Here's how the part is built. I have some questions about the finished solid (model axes, mm). A direction names the side the tool comes from. Round coordinates to 2 decimals unless told otherwise and drop trailing zeros. Write each loop counter-clockwise with the first axis right and the second up, starting at its lowest first coordinate (ties: lowest second). Pieces come first, ordered by that corner, then holes. Notation, with made-up numbers: (50, 28.25) -> (99, 28.25) arc R16 cw to (99, 32.25) -> close; hole circle Ø9 at (81.25, 34.25). An arc over 180 degrees is marked (long way). Put each result on its own line as item: value. Start each with the question number.
1. Suppose I cut it at C-C (x = 0). Please give me the cut outline in (y, z), then the cut area to 3 significant figures.
2. Suppose I cut it at D-D (x = 4). Please give me the cut outline in (y, z), then the cut area to 3 significant figures.
3. Suppose I cut it at B-B (y = 2.75). Please give me the cut outline in (x, z), then the cut area to 3 significant figures.
4. We'd pull the mould along Y, two halves only. Please class faces 4 (the face through (0.07, 2.95, 29.48)), 5 (the face through (5, 0.7, 22)), 6 (the face through (2, 0, 14)), 7 (the face through (0.07, 5.77, 29.56)): +Y half, -Y half, draft (parallel to the pull), parting line (faces both ways), or undercut.
5. Suppose I cut it at A-A (z = 5). Please give me the cut outline in (x, y).
6. For pin 1 (4 mm diameter, centred on x = -3, y = 6, fed in from +Z); pin 2 (5 mm diameter, centred on x = 0, z = 15, fed in from +Y), each with a flat end and sliding along its axis, tell me the tip position at first contact or that it passes through.
7. I need wall thicknesses on probe 1 along X at (y, z) = (0.3, 5); probe 2 along Y at (x, z) = (0.5, 12); probe 3 along Z at (x, y) = (-3.75, 5.25). Which ranges of each line are inside material? Lowest first, please. Write a range as from..to.
8. Which directions (+Z, -Z, +X, -X, +Y, -Y) give clear straight access to the entire face, cutting with the end or side of a thin tool? Please do faces 1 (the face through (0.07, 2.951, 35.613)), 2 (the face through (0, 0.5, 0)), 3 (the face through (0.07, 2.829, 28.486)).
```python
from build123d import *

# Parameters (mm, degrees)
EXTRUDE_THIN1_DEPTH = 5
FILLET1_R           = 3
SKETCH2_R           = 1.5
CUT_EXTRUDE1_DEPTH  = 10


with BuildPart() as part:
    # Sketch1 → Extrude-Thin1 (new, symmetric)
    with BuildSketch(Plane(origin=(0, 0, 0), x_dir=(0, 0, -1), z_dir=(1, 0, 0))):
        with BuildLine():
            Line((0, 0), (-28.808246407, 0))
            ThreePointArc((-28.808246407, 0), (-29.574290851, 0.35721239), (-29.79305416, 1.173648178))
            Line((-29.79305416, 1.173648178), (-29.156852475, 4.781727229))
            ThreePointArc((-29.156852475, 4.781727229), (-29.568083792, 5.774527451), (-30.641660228, 5.821400811))
            Line((-30.641660228, 5.821400811), (-40.724622204, 0))
            Line((-40.724622204, 0), (-41.224622204, 0.866025404))
            Line((-41.224622204, 0.866025404), (-31.141660228, 6.687426215))
            ThreePointArc((-31.141660228, 6.687426215), (-28.994507355, 6.593679496), (-28.172044722, 4.608079052))
            Line((-28.172044722, 4.608079052), (-28.808246407, 1))
            Line((-28.808246407, 1), (0, 1))
            Line((0, 1), (0, 0))
        make_face()
    extrude(amount=EXTRUDE_THIN1_DEPTH, both=True)

    # Fillet1
    fillet1_edges = [part.edges().sort_by_distance(p)[0] for p in [
        (-5, 0.433012702, 40.974622204),
        (5, 0.5, 0),
        (5, 0.433012702, 40.974622204),
        (-5, 0.5, 0),
    ]]
    fillet(fillet1_edges, radius=FILLET1_R)

    # Sketch2 → Cut-Extrude1 (cut)
    with BuildSketch(Plane(origin=(0, 1, 0), x_dir=(1, 0, 0), z_dir=(0, 1, 0))):
        with Locations(Location((0, -5, 0), (0, 0, 270))):
            Circle(SKETCH2_R)
        with Locations(Location((0, -15, 0), (0, 0, 270))):
            Circle(SKETCH2_R)
    extrude(amount=-CUT_EXTRUDE1_DEPTH, mode=Mode.SUBTRACT)


solid = part.part
```
Verdict:
1. outline: (0, 0) -> (1, 0) -> (1, 3.5) -> (0, 3.5) -> close; (0, 6.5) -> (1, 6.5) -> (1, 13.5) -> (0, 13.5) -> close; (0, 16.5) -> (1, 16.5) -> (1, 28.81) -> (4.61, 28.17) arc R2 ccw to (6.69, 31.14) -> (0.87, 41.22) -> (0, 40.72) -> (5.82, 30.64) arc R1 cw to (4.78, 29.16) -> (1.17, 29.79) arc R1 ccw to (0, 28.81) -> close
1. area: 42.4 mm^2
2. outline: (0, 0.76) -> (1, 0.76) -> (1, 28.81) -> (4.61, 28.17) arc R2 ccw to (6.69, 31.14) -> (1.25, 40.56) -> (0.38, 40.06) -> (5.82, 30.64) arc R1 cw to (4.78, 29.16) -> (1.17, 29.79) arc R1 ccw to (0, 28.81) -> close
2. area: 46.9 mm^2
3. outline: (-5, 28.5) -> (5, 28.5) -> (5, 29.52) -> (-5, 29.52) -> close; (-5, 35.96) -> (5, 35.96) -> (5, 37.96) -> (-5, 37.96) -> close
3. area: 30.2 mm^2
4. face 4: undercut
4. face 5: draft
4. face 6: -Y half
4. face 7: undercut
5. outline: (-5, 0) -> (-1.5, 0) -> (-1.5, 1) -> (-5, 1) -> close; (1.5, 0) -> (5, 0) -> (5, 1) -> (1.5, 1) -> close
6. pin 1: stops at z = 35.8
6. pin 2: stops at y = 1
7. probe 1: x = -5..-1.5, 1.5..5
7. probe 2: y = 0..1
7. probe 3: z = 28.16..29.19, 31.63..33.63
8. face 1: +X, -X, -Y
8. face 2: -Z, +X, -X, +Y, -Y
8. face 3: -Z, +X, -X
